Job drawing, mm, ordinate dimensions from the low corner. One solid piece. Round coordinates to 2 decimals unless told otherwise and drop trailing zeros. Write each loop counter-clockwise with the first axis right and the second up, starting at its lowest first coordinate (ties: lowest second). Pieces come first, ordered by that corner, then holes. Notation, with made-up numbers: (-16.5, 30.5) - (-6.5, 30.5) arc R24 cw to (-6.5, 66.5) - close; hole circle Ø6 at (-31, 76). An arc over 180 degrees is marked (long way). Write each question's results on one line, items separated by ' | '.
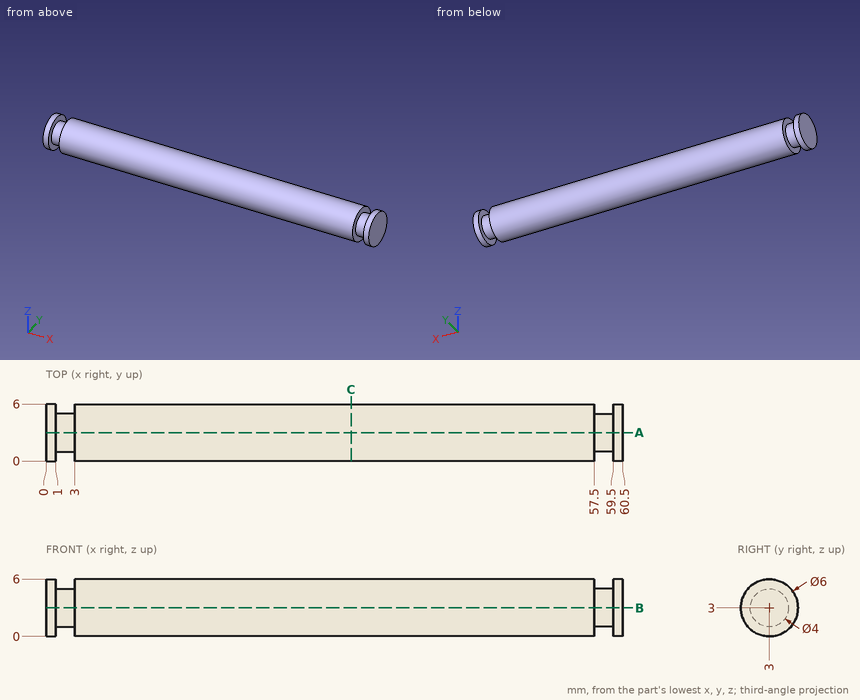
(1) Slice it at C-C, the plane x = 32. Write the cut outline in (y, z), and give its area (3 significant figures).
Worked answers:
outline: circle Ø6 at (3, 3) | area: 28.3 mm2
(2) Flat gauge pins, fed straight in: pin 1 Ø2 at (x, y) = (50.5, 5) entering from -Z; pin 2 Ø1.5 at (x, z) = (23, 4.5) entering from +Y. Where does each tip first touch, or does it go through?
Worked answers:
pin 1: stops at z = 0.17 | pin 2: stops at y = 5.9
(3) Drill centre lines: probe 1 along X at (y, z) = (1.55, 1.3); probe 2 along Y at (x, z) = (46, 2.9); probe 3 along Z at (x, y) = (23, 0.65). Where is each one in solid material? Low to high. Write a range as [from, to].
Worked answers:
probe 1: x = [0, 1], [3, 57.5], [59.5, 60.5] | probe 2: y = [0, 6] | probe 3: z = [1.14, 4.86]
(4) Slice it at A-A, the plane y = 3. Write the cut outline in (x, z), and give its area (3 significant figures).
Worked answers:
outline: (0, 0) - (1, 0) - (1, 1) - (3, 1) - (3, 0) - (57.5, 0) - (57.5, 1) - (59.5, 1) - (59.5, 0) - (60.5, 0) - (60.5, 6) - (59.5, 6) - (59.5, 5) - (57.5, 5) - (57.5, 6) - (3, 6) - (3, 5) - (1, 5) - (1, 6) - (0, 6) - close | area: 355 mm2
